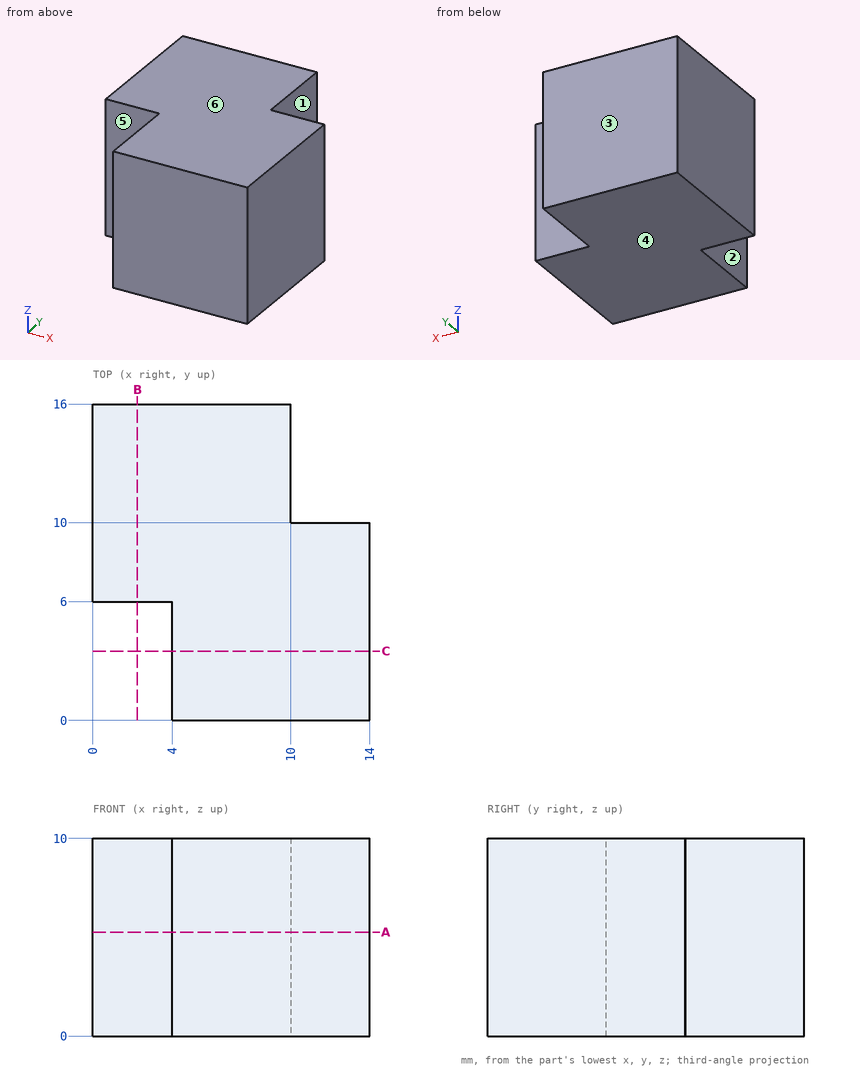
Design review of the part shown in the three views and the two pictorial views. Dimensions are in mm from the part's minimum x, y and z. A direction names the side the tool comes from. Give positions to 0.01 mm unless a question says otherwise; leave off trailing zeros. Write each loop counter-clockwise with the first axis right and the second up, starting at its lowest first coordinate (ties: lowest second). Pieces come first, ordered by that corner, then holes. Notation, with made-up numbers: M 58.5,-6 L 63.5,-6 A18 ccw 63.5,9 Z; hole C 28,-11 d3. An arc over 180 degrees is marked long. One line per item, written item: value.
1) For line 1 (X direction, y = 15.25, z = 6); line 2 (X direction, y = 5.5, z = 7.5), list the stretches that pass through material, from the lowest coordinate up. Write a range as from..to.
Results are:
line 1: x = 0..10
line 2: x = 4..14
2) The part is to be moulded in two halves that separate along Z. For the marked faces 4, 5 and 6, say which applies: +Z half, -Z half, draft (parallel to the pull), parting line (faces both ways), or undercut.
Results are:
face 4: -Z half
face 5: draft
face 6: +Z half
3) For the marked faces 1, 2 and 3, list the 3-axis set-ups (+Z, -Z, +X, -X, +Y, -Y) from which the entire face can be reached by the end or side of a thin tool; tool diameter is ignored.
Results are:
face 1: +Z, -Z, +X, +Y
face 2: +Z, -Z, -X, -Y
face 3: +Z, -Z, +X, -X, +Y
4) Take a section at B-B, the plane x = 2.25. Write out the cut boundary in (y, z), then the cut area to 3 significant figures.
Results are:
outline: M 6,0 L 16,0 L 16,10 L 6,10 Z
area: 100 mm²
5) Take a section at A-A, the plane z = 5.25. Write out the cut boundary in (x, y), then the cut area to 3 significant figures.
Results are:
outline: M 0,6 L 4,6 L 4,0 L 14,0 L 14,10 L 10,10 L 10,16 L 0,16 Z
area: 176 mm²
6) Take a section at C-C, the plane y = 3.5. Write out the cut boundary in (x, z).
Results are:
outline: M 4,0 L 14,0 L 14,10 L 4,10 Z
7) For P1, Ø2, axis at x = 1.5, z = 7, coming from the -Y side; P2, Ø5, axis at y = 2.5, z = 4.5, coming from the -X side, all flat-tipped, find the tip position at first contact; note any pin that passes through.
Results are:
P1: stops at y = 6
P2: stops at x = 4
